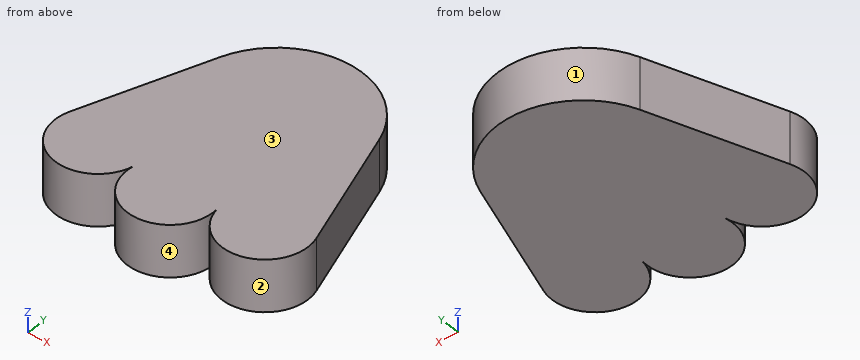
```python
from build123d import *

# Parameters (mm, degrees)
SALIENTE_EXTRUIR1_DEPTH = 3


with BuildPart() as part:
    # Croquis1 → Saliente-Extruir1 (new body)
    with BuildSketch(Plane.XY):
        with BuildLine():
            Line((-4.727593517, 4.627838916), (-7.301146697, -2.846311758))
            ThreePointArc((-7.301146697, -2.846311758), (-5.543839597, -6.085549813), (-2.468674969, -4.054748512))
            ThreePointArc((-2.468674969, -4.054748512), (0, -6.949265807), (2.468674969, -4.054748512))
            ThreePointArc((2.468674969, -4.054748512), (5.543839597, -6.085549813), (7.301146697, -2.846311758))
            Line((7.301146697, -2.846311758), (4.727593517, 4.627838916))
            ThreePointArc((4.727593517, 4.627838916), (0, 8), (-4.727593517, 4.627838916))
        make_face()
    extrude(amount=SALIENTE_EXTRUIR1_DEPTH)


solid = part.part
```
Geometry check sheet. Reference: the model listing, model coordinates, mm. Face numbers are marked on the shaded views. Coordinates: 2 decimals unless noted, no trailing zeros. Order: outer loops, then holes, each group sorted by start corner. A loop starts at its lowest first (then second) coordinate and runs counter-clockwise, first axis right, second up.
Item 1: Section check A-A (z = 0.2). Enter the section's corners in (x, y).
Item 2: Section check C-C (y = 5.25). Enter the section's corners in (x, z).
Item 3: Scan lines: line 1 along X through (y, z) = (4, 2.35); line 2 along Y through (x, z) = (2.75, 0.9); line 3 along Y through (x, z) = (4, 2.9). Record each from-to range of solid material in increasing order.
Item 4: Mould release check, pull along X, two halves, no side actions. Record for the marked faces 1, 2, 3 and 4: released by +X, released by -X, zero draft, split by the parting line, or undercut.
Item 5: Section check B-B (x = 5). Enter the section's corners in (y, z), plus the area to 3 significant figures.
Check sheet entries:
1. outline: (-7.3, -2.85) arc R2.5 ccw (long way) to (-2.47, -4.05) arc R2.5 ccw (long way) to (2.47, -4.05) arc R2.5 ccw (long way) to (7.3, -2.85) - (4.73, 4.63) arc R5 ccw to (-4.73, 4.63) - close
2. outline: (-4.47, 0) - (4.47, 0) - (4.47, 3) - (-4.47, 3) - close
3. line 1: x = -4.94 to 4.94
3. line 2: y = -4.87 to 7.18
3. line 3: y = -5.98 to 6
4. face 1: split by the parting line
4. face 2: undercut
4. face 3: zero draft
4. face 4: undercut
5. outline: (-6.16, 0) - (3.84, 0) - (3.84, 3) - (-6.16, 3) - close
5. area: 30.0 mm2
